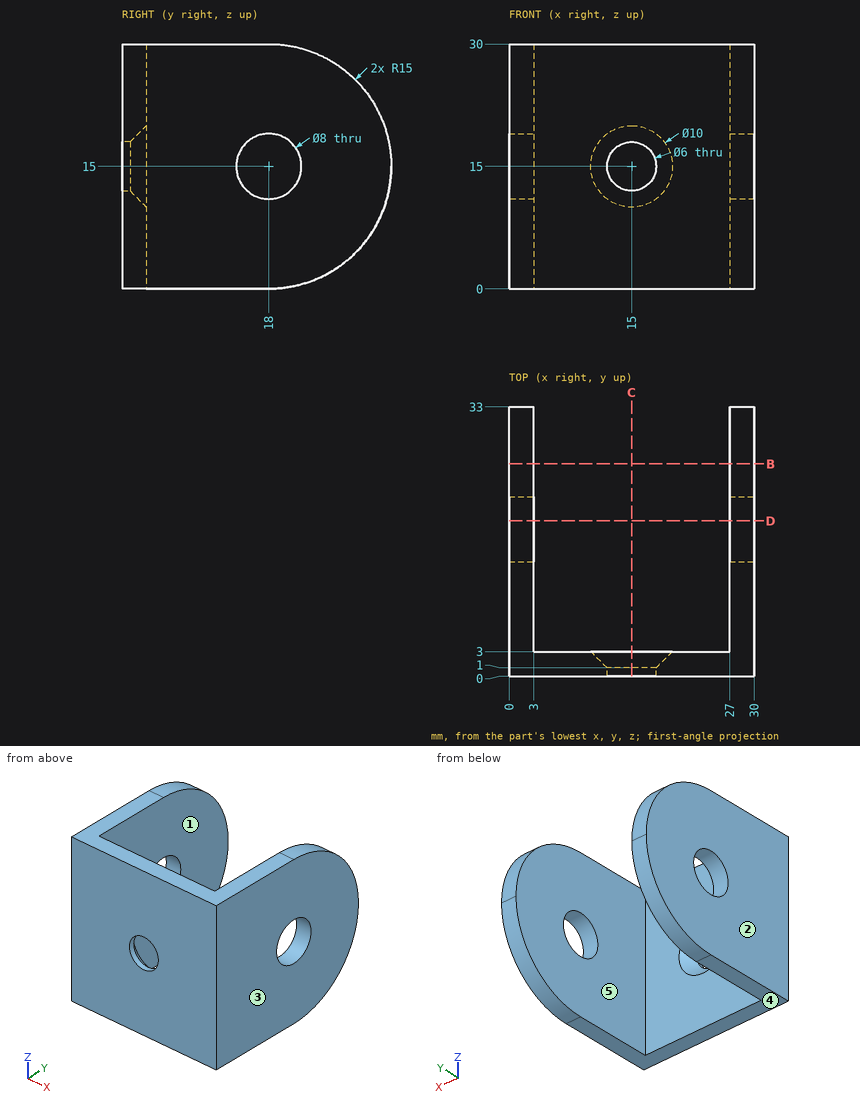
Study the drawing (mm; zero at the part's minimum x, y, z) and answer. A direction names the side the tool comes from. Coordinates: 2 decimals unless noted, no trailing zeros. Write each loop counter-clockwise with the first axis right and the second up, starting at its lowest first coordinate (ties: lowest second). Pieces come first, ordered by that corner, then holes.
Q1. Section C-C, the plane x = 15 is taken. Write down the section's boundary in (y, z), then the cut area to 3 significant figures.
Returned:
outline: (0, 0) - (3, 0) - (3, 10) - (1, 12) - (0, 12) - close; (0, 18) - (1, 18) - (3, 20) - (3, 30) - (0, 30) - close
area: 68.0 mm2
Q2. Section D-D, the plane y = 19 is taken. Write down the section's boundary in (x, z), then the cut area to 3 significant figures.
Returned:
outline: (0, 0.03) - (3, 0.03) - (3, 11.13) - (0, 11.13) - close; (0, 18.87) - (3, 18.87) - (3, 29.97) - (0, 29.97) - close; (27, 0.03) - (30, 0.03) - (30, 11.13) - (27, 11.13) - close; (27, 18.87) - (30, 18.87) - (30, 29.97) - (27, 29.97) - close
area: 133 mm2
Q3. Which of the six approach directions +Z, -Z, +X, -X, +Y, -Y give full straight-line access (tool end or side, diameter ignored) to the marked faces 1 and 2?
Returned:
face 1: +Z, -Z, +Y
face 2: +Z, -Z, -X, +Y, -Y
Q4. Section B-B, the plane y = 26 is taken. Write down the section's boundary in (x, z), then the cut area to 3 significant figures.
Returned:
outline: (0, 2.31) - (3, 2.31) - (3, 27.69) - (0, 27.69) - close; (27, 2.31) - (30, 2.31) - (30, 27.69) - (27, 27.69) - close
area: 152 mm2
Q5. The mould has two halves that part along X. Classify the marked faces 3, 4 and 5: released by +X, released by -X, zero draft, split by the parting line, or undercut.
Returned:
face 3: released by +X
face 4: zero draft
face 5: undercut
Q6. Find the intervals of material crossed by line 1 along X through (y, z) = (0.6, 15); line 2 along X through (y, z) = (14.5, 9.5); line 3 along Y through (x, z) = (0.95, 15), in increasing order.
Returned:
line 1: x = 0 to 12, 18 to 30
line 2: x = 0 to 3, 27 to 30
line 3: y = 0 to 14, 22 to 33
